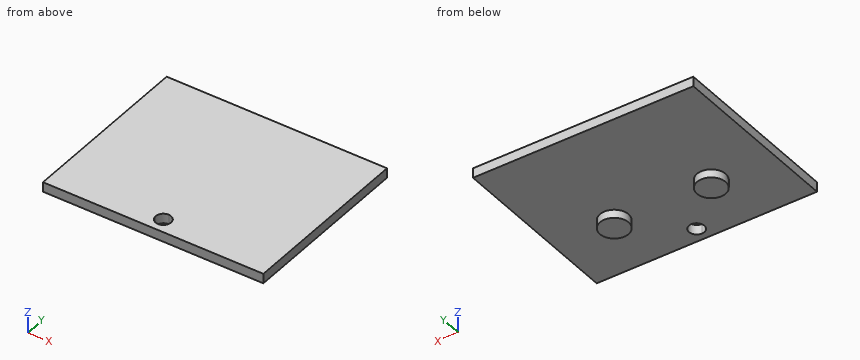
from build123d import *

# Parameters (mm, degrees)
SKETCH_1_W          = 45.4
SKETCH_1_H          = 36.5
EXTRUDE_1_DEPTH     = 2
CUT_EXTRUDE_9_DEPTH = 85.579435184
SKETCH_10_3_R       = 2.95
EXTRUDE_3_DEPTH     = 1.7


with BuildPart() as part:
    # Sketch 1 → Extrude 1 (new body)
    with BuildSketch(Plane.XY):
        with Locations((-49.741035857, 25.361663348)):
            Rectangle(SKETCH_1_W, SKETCH_1_H)
    extrude(amount=EXTRUDE_1_DEPTH)

    # Sketch 10 → Cut-Extrude 9 (cut, through all)
    with BuildSketch(Plane(origin=(0, 0, 0), x_dir=(-1, 0, 0), z_dir=(0, 0, -1))):
        with BuildLine():
            ThreePointArc((51.341035857, 10.111663348), (50.872406706, 11.243034198), (49.741035857, 11.711663348))
            Line((49.741035857, 11.711663348), (49.741035857, 8.511663348))
            ThreePointArc((49.741035857, 8.511663348), (50.872406706, 8.980292499), (51.341035857, 10.111663348))
        make_face()
        with BuildLine():
            Line((49.741035857, 8.511663348), (49.741035857, 11.711663348))
            ThreePointArc((49.741035857, 11.711663348), (48.141035857, 10.111663348), (49.741035857, 8.511663348))
        make_face()
    extrude(amount=-CUT_EXTRUDE_9_DEPTH, mode=Mode.SUBTRACT)

    # Sketch 10_3 → Extrude 3 (add)
    with BuildSketch(Plane(origin=(0, 0, 0), x_dir=(-1, 0, 0), z_dir=(0, 0, -1))):
        with Locations((59.741035857, 20.111663348)):
            Circle(SKETCH_10_3_R)
        with Locations(Location((39.741035857, 20.111663348, 0), (0, 0, 180))):
            Circle(SKETCH_10_3_R)
    extrude(amount=EXTRUDE_3_DEPTH)


solid = part.part
Could you check a few things on this model? Use its own coordinates, in mm. Coordinates: 2 decimals unless noted, no trailing zeros. Order: outer loops, then holes, each group sorted by start corner. A loop starts at its lowest first (then second) coordinate and runs counter-clockwise, first axis right, second up.
Q1. Will this pin go through, and if not, where does the flat tip stop? pin 1 (11 mm diameter, centred on x = -58.5, y = 31, fed in from -Z).
Q2. Please list where these lines run through material, in increasing order: L1, parallel to Y at x = -40, z = -1; L2, parallel to Z at x = -54, y = 25; L3, parallel to X at y = 21.5, z = -0.9.
Q3. Suppose I cut it at D-D on x = -40.5. Please give me the cut outline in (y, z), and give its area (3 significant figures).
Q4. Suppose I cut it at B-B on x = -55. Please give me the cut outline in (y, z).
Q5. Suppose I cut it at C-C on z = -1.15. Please give me the cut outline in (x, y), and give its area (3 significant figures).
Q6. Suppose I cut it at A-A on y = 33.5. Please give me the cut outline in (x, z).
Answer:
1. pin 1: stops at z = 0
2. L1: y = 17.17 to 23.05
2. L2: z = 0 to 2
2. L3: x = -62.34 to -57.14, -42.34 to -37.14
3. outline: (7.11, 0) - (17.26, 0) - (17.26, -1.7) - (22.96, -1.7) - (22.96, 0) - (43.61, 0) - (43.61, 2) - (7.11, 2) - close
3. area: 82.7 mm2
4. outline: (7.11, 0) - (43.61, 0) - (43.61, 2) - (7.11, 2) - close
5. outline: circle Ø5.9 at (-59.74, 20.11); circle Ø5.9 at (-39.74, 20.11)
5. area: 54.7 mm2
6. outline: (-72.44, 0) - (-27.04, 0) - (-27.04, 2) - (-72.44, 2) - close
